from build123d import *

# Parameters (mm, degrees)
F0_W     = 25.4
F0_H     = 6.35
F1_DEPTH = 12.7


with BuildPart() as f1:
    # F0 (on Top) → F1 (new body)
    with BuildSketch(Plane.XY):
        with BuildLine():
            Line((0, 0), (0, 25.4))
            ThreePointArc((0, 25.4), (-9.518756, 9.518756), (-25.4, 0))
            Line((-25.4, 0), (0, 0))
        make_face()
        Polygon((12.7, 25.4), (0, 25.4), (0, 0), (0, -6.35), (12.7, -6.35), align=None)
        with Locations((-12.7, -3.175)):
            Rectangle(F0_W, F0_H)
    extrude(amount=F1_DEPTH)


solid = f1.part
The model under review builds one solid part; all positions refer to its coordinate system, in mm. Give positions to 0.01 mm unless a question says otherwise; leave off trailing zeros. Order: outer loops, then holes, each group sorted by start corner. A loop starts at its lowest first (then second) coordinate and runs counter-clockwise, first axis right, second up. Notation, with made-up numbers: (-26.5, -5.5) -> (6.5, -5.5) arc R20 ccw to (6.5, 20.5) -> close; hole circle Ø5 at (-10.5, 63). An arc over 180 degrees is marked (long way). Write item = value, one per line. Start each with the question number.
(1) Take a section at A-A (z = 3). Write out the cut boundary in (x, y).
(2) For pin 1 Ø2 at (x, z) = (-13.5, 11) entering from +Y, flat-tipped, find the tip position at first contact; note if it passes through.
(3) For L1, parallel to Y at x = -15, z = 6; L2, parallel to Y at x = -23, z = 8.5; L3, parallel to X at y = 2.5, z = 11.75, list the stretches that pass through material, from the lowest coordinate up. Write a range as from..to.
(4) Draft analysis for pull direction Z (two halves, no side actions). For faces 1 (the flat face through (12.7, 9, 6)), 2 (the flat face through (-2, 6, 0)), 3 (the flat face through (-2, 6, 12.7)), state which applies: +Z half, -Z half, draft (parallel to the pull), parting line (faces both ways), or undercut.
(5) Take a section at B-B (x = -19.5). Write out the cut boundary in (y, z), plus the area to 3 significant figures.
(6) Take a section at C-C (y = 9.5). Write out the cut boundary in (x, z).
Returned:
q1.outline = (-25.4, -6.35) -> (12.7, -6.35) -> (12.7, 25.4) -> (0, 25.4) arc R38.1 cw to (-25.4, 0) -> close
q2.pin_1 = 6.84
q3.L1 = -6.35..4.98
q3.L2 = -6.35..0.82
q3.L3 = -19.19..12.7
q4.face_1 = draft
q4.face_2 = -Z half
q4.face_3 = +Z half
q5.outline = (-6.35, 0) -> (2.34, 0) -> (2.34, 12.7) -> (-6.35, 12.7) -> close
q5.area = 110 mm²
q6.outline = (-9.54, 0) -> (12.7, 0) -> (12.7, 12.7) -> (-9.54, 12.7) -> close
